The model under review builds one solid part; all positions refer to its coordinate system, in mm. Round coordinates to 2 decimals unless told otherwise and drop trailing zeros. Loops run counter-clockwise (first coordinate to the right, second up) from the corner with the lowest first, then second, coordinate; pieces in that order, holes last. Notation, with made-up numbers: (55.5, 42) -> (75.5, 42) arc R18 ccw to (75.5, 50) -> close; hole circle Ø7 at (19, 60.5). An arc over 180 degrees is marked (long way). Use a Markdown table: item, result. Add a question column.
1) Insertion check: pin 1 (5 mm diameter, centred on x = -53.71, z = 6.93, fed in from +Y). The pin has a flat end and moves straight along its axis. Give the tip position at first contact, or say it passes through.
2) Wall thickness on probe 1 along X at (y, z) = (-2.5, -1.5); probe 2 along X at (y, z) = (-0.4, -4.5); probe 3 along Z at (x, y) = (-56.5, -1.8): over which ranges is each line inside the solid? List them lowest first.
3) Consider section B-B on y = -3. Give the boundary of the cut face in (x, z) (3 decimals), plus the area to 3 significant figures.
4) Consider section A-A on x = -19.05. Give the boundary of the cut face in (y, z) (3 decimals).
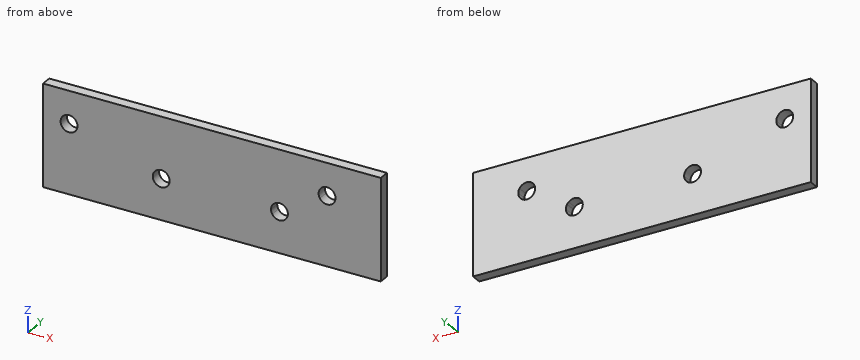
from build123d import *

# Parameters (mm, degrees)
F1_DEPTH = 3.96875


with BuildPart() as f1:
    # F0 (on Front) → F1 (new body)
    with BuildSketch(Plane.XZ):
        with BuildLine():
            Line((46.0279571805, 8.5667743083), (63.5, 19.05))
            Line((63.5, 19.05), (45.9832364526, 19.05))
            Line((45.9832364526, 19.05), (27.5244896752, -1.4505151791))
            ThreePointArc((27.5244896752, -1.4505151791), (27.8505466804, -1.7912266182), (28.1225400391, -2.1764759765))
            Line((28.1225400391, -2.1764759765), (40.5828771022, 5.2997262613))
            ThreePointArc((40.5828771022, 5.2997262613), (41.6718931179, 9.6557903239), (46.0279571805, 8.5667743083))
        make_face()
        with BuildLine():
            Line((27.5244896752, -1.4505151791), (45.9832364526, 19.05))
            Line((45.9832364526, 19.05), (-63.5, 19.05))
            Line((-63.5, 19.05), (-63.5, -19.05))
            Line((-63.5, -19.05), (0, -19.05))
            Line((0, -19.05), (0, -9.525))
            Line((0, -9.525), (-15.9821089289, -4.6277220653))
            ThreePointArc((-15.9821089289, -4.6277220653), (-19.9802006219, -6.8456797926), (-22.0493462104, -2.7685839881))
            ThreePointArc((-22.0493462104, -2.7685839881), (-18.5219371336, -0.6792214053), (-15.875, -3.81))
            Line((-15.875, -3.81), (0, -3.81))
            Line((0, -3.81), (22.225, -3.81))
            ThreePointArc((22.225, -3.81), (24.1086111582, -0.909493172), (27.5244896752, -1.4505151791))
        make_face()
        with BuildLine():
            ThreePointArc((-50.535970122, 6.9332502848), (-50.5709933433, 6.4629622568), (-50.6752903294, 6.0030496629))
            ThreePointArc((-50.6752903294, 6.0030496629), (-56.8509469007, 7.4035383128), (-50.535970122, 6.9332502848))
        make_face(mode=Mode.SUBTRACT)
        with BuildLine():
            Line((63.5, -19.05), (63.5, 19.05))
            Line((63.5, 19.05), (46.0279571805, 8.5667743083))
            ThreePointArc((46.0279571805, 8.5667743083), (46.3652120384, 7.7807644073), (46.4804171413, 6.9332502848))
            ThreePointArc((46.4804171413, 6.9332502848), (44.1529312639, 3.8734553877), (40.5828771022, 5.2997262613))
            Line((40.5828771022, 5.2997262613), (28.1225400391, -2.1764759765))
            ThreePointArc((28.1225400391, -2.1764759765), (28.4597948971, -2.9624858775), (28.575, -3.81))
            ThreePointArc((28.575, -3.81), (26.2475141225, -6.8697948971), (22.6774599609, -5.4435240235))
            Line((22.6774599609, -5.4435240235), (10.5083445014, -12.7449932991))
            Line((10.5083445014, -12.7449932991), (0, -19.05))
            Line((0, -19.05), (63.5, -19.05))
        make_face()
        Polygon((0, -9.525), (0, -19.05), (10.5083445014, -12.7449932991), align=None)
        with BuildLine():
            ThreePointArc((22.6774599609, -5.4435240235), (22.3402051029, -4.6575141225), (22.225, -3.81))
            Line((22.225, -3.81), (0, -3.81))
            Line((0, -3.81), (-15.875, -3.81))
            ThreePointArc((-15.875, -3.81), (-15.9018911113, -4.222353519), (-15.9821089289, -4.6277220653))
            Line((-15.9821089289, -4.6277220653), (0, -9.525))
            Line((0, -9.525), (10.5083445014, -12.7449932991))
            Line((10.5083445014, -12.7449932991), (22.6774599609, -5.4435240235))
        make_face()
    extrude(amount=F1_DEPTH)


solid = f1.part
Result set:
| question | item | result |
|---|---|---|
| 1 | pin 1 | through |
| 2 | probe 1 | -63.5 to -21.23, -16.87 to 23.22, 27.58 to 63.5 |
| 2 | probe 2 | -63.5 to -22.15, -15.95 to 22.3, 28.5 to 63.5 |
| 2 | probe 3 | -19.05 to 5.42, 8.45 to 19.05 |
| 3 | outline | (-63.5, -19.05) -> (63.5, -19.05) -> (63.5, 19.05) -> (-63.5, 19.05) -> close; hole circle Ø6.35 at (-53.711, 6.933); hole circle Ø6.35 at (-19.05, -3.81); hole circle Ø6.35 at (25.4, -3.81); hole circle Ø6.35 at (43.305, 6.933) |
| 3 | area | 4,710 mm2 |
| 4 | outline | (-3.969, -19.05) -> (0, -19.05) -> (0, -6.985) -> (-3.969, -6.985) -> close; (-3.969, -0.635) -> (0, -0.635) -> (0, 19.05) -> (-3.969, 19.05) -> close |
